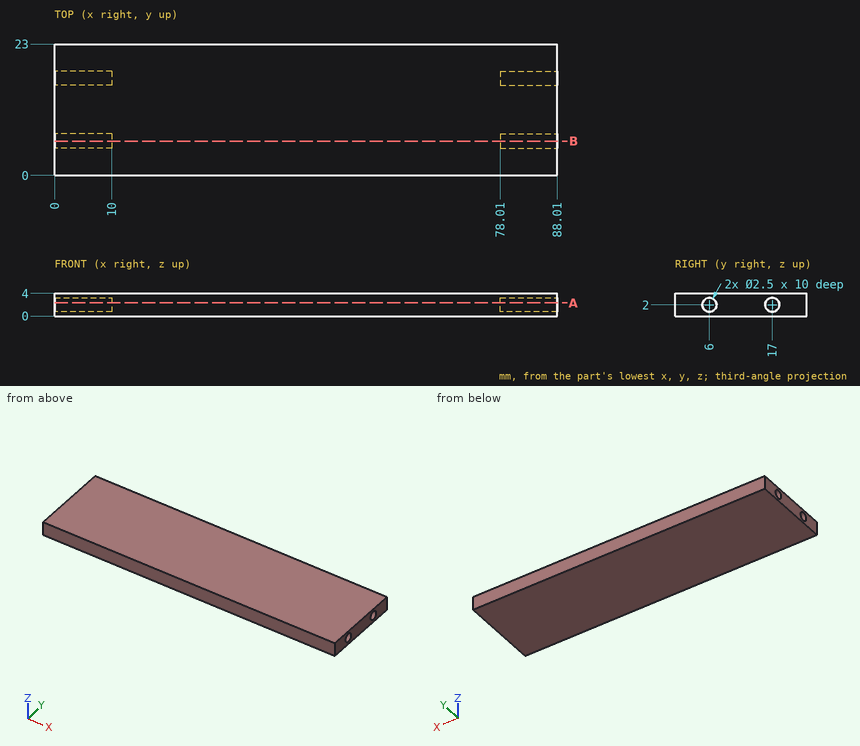
Study the drawing (mm; zero at the part's minimum x, y, z) and answer. Coordinates: 2 decimals unless noted, no trailing zeros. Write each loop counter-clockwise with the first axis right and the second up, starting at its lowest first coordinate (ties: lowest second). Pieces come first, ordered by that corner, then holes. Notation, with made-up numbers: (24.5, -6) - (34.5, -6) arc R9 ccw to (34.5, 4) - close; hole circle Ø8 at (76.5, 64). An arc over 180 degrees is marked (long way). Put each result on its own line as item: value.
1. The part is cut by section B-B on y = 6. Give the vertices of the cut face in (x, z).
Answer sheet:
outline: (0, 0) - (88.01, 0) - (88.01, 0.75) - (78.01, 0.75) - (78.01, 3.25) - (88.01, 3.25) - (88.01, 4) - (0, 4) - (0, 3.25) - (10, 3.25) - (10, 0.75) - (0, 0.75) - close
2. Find the intervals of material crossed by line 1 along Y through (x, z) = (5.25, 2); line 2 along X through (y, z) = (6.75, 1.4); line 3 along Y through (x, z) = (84.5, 1.1), in increasing order. Write a range as from..to.
Answer sheet:
line 1: y = 0..4.75, 7.25..15.75, 18.25..23
line 2: x = 10..78.01
line 3: y = 0..5.13, 6.87..16.13, 17.87..23
3. The part is cut by section A-A on z = 2.35. Give the vertices of the cut face in (x, y), plus the area to 3 significant figures.
Answer sheet:
outline: (0, 0) - (88.01, 0) - (88.01, 4.8) - (78.01, 4.8) - (78.01, 7.2) - (88.01, 7.2) - (88.01, 15.8) - (78.01, 15.8) - (78.01, 18.2) - (88.01, 18.2) - (88.01, 23) - (0, 23) - (0, 18.2) - (10, 18.2) - (10, 15.8) - (0, 15.8) - (0, 7.2) - (10, 7.2) - (10, 4.8) - (0, 4.8) - close
area: 1,930 mm^2
4. Flat-ended cylindrical pins translate along their axes: pin 1 Ø2 at (y, z) = (17, 2) entering from +X; pin 2 Ø0.8 at (y, z) = (6, 1.5) entering from -X. Find the tip coordinate at first contact, or state that the pin passes through.
Answer sheet:
pin 1: stops at x = 78.01
pin 2: stops at x = 10
